Geometry check sheet. Reference: the model listing, model coordinates, mm. Coordinates: 2 decimals unless noted, no trailing zeros. Order: outer loops, then holes, each group sorted by start corner. A loop starts at its lowest first (then second) coordinate and runs counter-clockwise, first axis right, second up. Notation, with made-up numbers: (-31.75, 31.25) - (-16.75, 31.25) arc R14 ccw to (-16.75, 52.25) - close; hole circle Ø1 at (69.5, -10.5). An arc over 180 degrees is marked (long way). Return JSON: item names as keys, results as strings. Group by question number.
Item 1: Section check B-B on x = 0. Enter the section's corners in (y, z), then the cut area to 3 significant figures.
Item 2: Section check C-C on x = 20. Enter the section's corners in (y, z).
Item 3: Scan lines: probe 1 along Z at (x, y) = (0, 1.9); probe 2 along Z at (x, y) = (-7, 3.25); probe 3 along X at (y, z) = (4.2, 3.5). Record each from-to range of solid material in increasing order.
Item 4: Section check D-D on z = 22. Enter the section's corners in (x, y).
Item 5: Section check A-A on y = 1. Give the number of separate pieces and of enclosed holes in the cut face, then the cut area to 3 significant figures.
Item 6: Gauge pin test, flat ends, axial feed: pin 1 (1.5 mm diameter, centred on y = 2.5, z = 44, fed in from -X); pin 2 (1 mm diameter, centred on y = 3, z = 29, fed in from +X); pin 3 (8.5 mm diameter, centred on x = 0, z = 0, fed in from -Y); pin 4 (3 mm diameter, centred on x = 35, y = 4.5, fed in from -Z). Record the tip position at first contact, or that the pin passes through.
from build123d import *

# Parameters (mm, degrees)
SKETCH1_R               = 12.5
BOSS_EXTRUDE1_DEPTH     = 5
EXTRUDE_THIN1_DEPTH     = 5
SKETCH6_W               = 56.5
SKETCH6_H               = 12.459935794
BOSS_EXTRUDE3_DEPTH     = 5
CUT_EXTRUDE3_DEPTH      = 80.717487022
CUT_EXTRUDE3_DEPTH_BACK = 80.717487022
SKETCH7_R               = 3.25
CUT_EXTRUDE_THIN1_START = -5
CUT_EXTRUDE_THIN1_DEPTH = 85.717487022
FILLET1_R               = 2.075
FILLET2_R               = 4
BOSS_EXTRUDE4_DEPTH     = 5
SKETCH9_4_W             = 9.626496109
SKETCH9_4_H             = 23.122525611
CUT_EXTRUDE5_DEPTH      = 81.602542459


with BuildPart() as part:
    # Sketch1 → Boss-Extrude1 (new body)
    with BuildSketch(Plane(origin=(0, 0, 0), x_dir=(1, 0, 0), z_dir=(0, 1, 0))):
        with Locations(Location((0, 0, 0), (0, 0, 270))):
            Circle(SKETCH1_R)
    extrude(amount=BOSS_EXTRUDE1_DEPTH)



with BuildPart() as body_2:
    # Sketch4 → Extrude-Thin1 (new body)
    with BuildSketch(Plane(origin=(0, 0, 0), x_dir=(1, 0, 0), z_dir=(0, 1, 0))):
        with BuildLine():
            ThreePointArc((16.811373022, -54.987523468), (46.221769485, -34.202310238), (57.5, 0))
            Line((57.5, 0), (42.5, 0))
            ThreePointArc((42.5, 0), (34.163916576, -25.279968437), (12.425797451, -40.642952128))
            Line((12.425797451, -40.642952128), (16.811373022, -54.987523468))
        make_face()
    extrude(amount=EXTRUDE_THIN1_DEPTH)


with BuildPart() as part_1:
    add(part.part)

    add(body_2.part)  # Boss-Extrude3 merges body 2
    # Sketch6 → Boss-Extrude3 (add)
    with BuildSketch(Plane(origin=(0, 0, 0), x_dir=(1, 0, 0), z_dir=(0, 1, 0))):
        with Locations((29.25, 6.229967897)):
            Rectangle(SKETCH6_W, SKETCH6_H)
    extrude(amount=BOSS_EXTRUDE3_DEPTH)

    # Sketch7 → Cut-Extrude3 (cut, two sides: drawn at the far end of the back side and taken through both)
    with BuildSketch(Plane(origin=(0, 5, 0), x_dir=(1, 0, 0), z_dir=(0, 1, 0)).offset(-CUT_EXTRUDE3_DEPTH_BACK)):
        with Locations(Location((0, 0, 0), (0, 0, 270))):
            Circle(SKETCH7_R)
    extrude(amount=CUT_EXTRUDE3_DEPTH + CUT_EXTRUDE3_DEPTH_BACK, mode=Mode.SUBTRACT)

    # Sketch8 → Cut-Extrude-Thin1 (cut)
    with BuildSketch(Plane(origin=(0, 5, 0), x_dir=(1, 0, 0), z_dir=(0, 1, 0)).offset(CUT_EXTRUDE_THIN1_START)):
        with BuildLine():
            ThreePointArc((-5.0375, 8.725205943), (-10.075, 0), (-5.0375, -8.725205943))
            Line((-5.0375, -8.725205943), (-2.9625, -5.131200517))
            ThreePointArc((-2.9625, -5.131200517), (-5.925, 0), (-2.9625, 5.131200517))
            Line((-2.9625, 5.131200517), (-5.0375, 8.725205943))
        make_face()
    cut_extrude_thin1 = extrude(amount=CUT_EXTRUDE_THIN1_DEPTH, mode=Mode.SUBTRACT)

    # Mirror2: Cut-Extrude-Thin1 across plane
    add(cut_extrude_thin1.mirror(Plane(origin=(0, 0, 0), x_dir=(0, 0, 1), z_dir=(1, 0, 0))), mode=Mode.SUBTRACT)

    # Fillet1
    fillet1_edges = [part_1.edges().sort_by_distance(p)[0] for p in [
        (2.9625, 2.5, -5.131200517),
        (5.0375, 2.5, -8.725205943),
        (-5.0375, 2.5, -8.725205943),
        (-2.9625, 2.5, -5.131200517),
        (2.9625, 2.5, 5.131200517),
        (5.0375, 2.5, 8.725205943),
        (-5.0375, 2.5, 8.725205943),
        (-2.9625, 2.5, 5.131200517),
    ]]
    fillet(fillet1_edges, radius=FILLET1_R - 0.0001)  # a hair under: the kernel refuses the full size

    # Fillet2
    fillet2_edges = [part_1.edges().sort_by_distance(p)[0] for p in [
        (42.5, 2.5, 0),
        (12.5, 2.5, 0),
        (57.5, 2.5, -12.459935794),
    ]]
    fillet(fillet2_edges, radius=FILLET2_R)

    # Sketch9 → Boss-Extrude4 (add)
    with BuildSketch(Plane(origin=(0, 0, 0), x_dir=(1, 0, 0), z_dir=(0, 1, 0))):
        with BuildLine():
            Line((16.811373022, -54.987523468), (14.618585236, -47.815237798))
            Line((14.618585236, -47.815237798), (14.618585236, -55.610673128))
            ThreePointArc((14.618585236, -55.610673128), (15.718067562, -55.309966119), (16.811373022, -54.987523468))
        make_face()
        with BuildLine():
            Line((14.618585236, -47.815237798), (12.425797451, -40.642952128))
            Line((12.425797451, -40.642952128), (11.862973877, -56.262952738))
            ThreePointArc((11.862973877, -56.262952738), (13.244795598, -55.953779046), (14.618585236, -55.610673128))
            Line((14.618585236, -55.610673128), (14.618585236, -47.815237798))
        make_face()
    extrude(amount=BOSS_EXTRUDE4_DEPTH)

    # Sketch9<4> → Cut-Extrude5 (cut, through all)
    with BuildSketch(Plane(origin=(0, 0, 0), x_dir=(1, 0, 0), z_dir=(0, 1, 0))):
        with Locations((9.805337182, -49.150976699)):
            Rectangle(SKETCH9_4_W, SKETCH9_4_H)
    extrude(amount=CUT_EXTRUDE5_DEPTH, mode=Mode.SUBTRACT)


solid = part_1.part
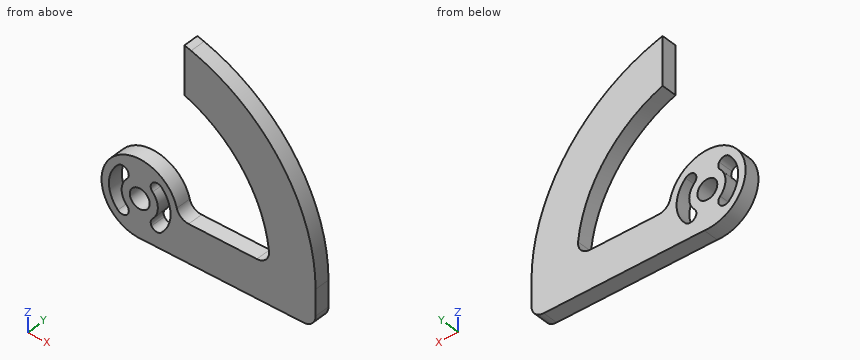
Computed:
{
 "1": {"outline": "(0, -12.5) - (5, -12.5) - (5, -3.25) - (0, -3.25) - close; (0, 3.25) - (5, 3.25) - (5, 12.5) - (0, 12.5) - close", "area": "92.5 mm²"},
 "2": {"outline": "(0, -12.46) - (5, -12.46) - (5, 0) - (0, 0) - close; (0, 37.5) - (5, 37.5) - (5, 53.91) - (0, 53.91) - close"},
 "3": {"probe 1": "z = -12.5 to -3.25, 3.25 to 12.5", "probe 2": "z = -10.36 to -7.24, 7.24 to 10.36", "probe 3": "x = -12 to -9.45, -4.78 to 4.78, 9.45 to 12, 42.26 to 57.39"},
 "4": {"outline": "(36.36, 0) - (53.12, 0) - (53.12, 5) - (36.36, 5) - close"},
 "5": {"separate pieces": "1", "enclosed holes": "3", "area": "1,880 mm²"},
 "6": {"pin 1": "stops at x = 14.62", "pin 2": "stops at x = 49.94", "pin 3": "stops at y = 0", "pin 4": "stops at z = -12.46"}
}
